from build123d import *

# Parameters (mm, degrees)
SKETCH001_W = 6
SKETCH001_H = 2
SKETCH002_R = 1.6
HOLE_DEPTH  = 2
HOLE_TIPS_R = 1.6


with BuildPart() as part:
    # AdditivePipe: sweep along a path in Sketch
    with BuildLine(Plane.XZ) as additivepipe_path:
        Line((-3, 0), (5.65, 0))
        ThreePointArc((5.65, 0), (6.053202, 0.204318), (6.126879, 0.650289))
        ThreePointArc((6.126879, 0.650289), (5.65, 3.75), (6.126879, 6.849711))
        ThreePointArc((6.126879, 6.849711), (6.053202, 7.295682), (5.65, 7.5))
        Line((5.65, 7.5), (2.5, 7.5))
        ThreePointArc((2.5, 7.5), (2.401942, 7.49029), (2.307692, 7.461538))
        ThreePointArc((2.307692, 7.461538), (0, 7), (-2.307692, 7.461538))
    # Sketch001 → AdditivePipe (sweep)
    with BuildSketch(Plane.YZ):
        with Locations((0, -1)):
            Rectangle(SKETCH001_W, SKETCH001_H)
    sweep(path=additivepipe_path.line)

    # Sketch002 (on DatumPlane) → Hole (cut)
    with BuildSketch(Plane.XY.offset(-2)):
        Circle(SKETCH002_R)
    extrude(amount=HOLE_DEPTH, mode=Mode.SUBTRACT)

    # Hole tips → Hole tip 1 section 0
    with BuildSketch(Plane.XY, mode=Mode.PRIVATE) as hole_tip_1_s0:
        Circle(HOLE_TIPS_R)
    loft([hole_tip_1_s0.sketch, Vertex(0, 0, 0.961377)], mode=Mode.SUBTRACT)


solid = part.part
Design review of the part built by this model. Coordinates are the model's own, in mm. A direction names the side the tool comes from. Give positions to 0.01 mm unless a question says otherwise; leave off trailing zeros. Write each loop counter-clockwise with the first axis right and the second up, starting at its lowest first coordinate (ties: lowest second). Pieces come first, ordered by that corner, then holes. Notation, with made-up numbers: M 2.25,37.5 L 32.25,37.5 A13 ccw 32.25,56.5 Z; hole C -28.5,53.25 d4. An arc over 180 degrees is marked long. Return JSON: item names as keys, results as strings. Group by question number.
Item 1: Take a section at B-B (x = 0). Give the boundary of the cut face in (y, z), plus the area to 3 significant figures.
Item 2: Take a section at A-A (y = 0). Give the boundary of the cut face in (x, z), plus the area to 3 significant figures.
Item 3: Wall thickness on line 1 along Y through (x, z) = (0, -1.1); line 2 along Z through (x, y) = (2.75, 1.5); line 3 along Y through (x, z) = (-0.75, -0.5): over which ranges is each line inside the solid? List them lowest first.
Item 4: The part is to be moulded in two halves that separate along Z. For faces 1 (the flat face through (2, 0, -2)), 2 (the cylindrical face through (-1.27, -0.97, -1.01)), 3 (the flat face through (4, 0, 7.5)), say which applies: pulls with the +Z half, pulls with the -Z half, needs draft (parallel to the pull), parting line crosses it, or undercut.
Item 5: Take a section at C-C (z = -1). Give the boundary of the cut face in (x, y), plus the area to 3 significant figures.
Item 6: Clearance check with a flat-ended pin moving along its axis: pin 1 Ø6 at (x, z) = (2.5, 0.5) entering from +Y. State where the tip first meets the part, or that it passes through.
Item 7: Tool access review of faces 4 (the flat face through (2, 0, 0)), 5 (the flat face through (-1.918, -0.042, 8.398)), 6 (the cylindrical face through (0, 0, 7)): name each direction out of +Z, -Z, +X, -X, +Y, -Y from which nothing blocks a thin tool from reaching the whole face with its end or side.
Item 8: Take a section at D-D (x = 2.75). Give the boundary of the cut face in (y, z), plus the area to 3 significant figures.
Return value:
{
 "1": {"outline": "M -3,-2 L -1.6,-2 L -1.6,0 L -3,0 Z; M -3,7 L 3,7 L 3,9 L -3,9 Z; M 1.6,-2 L 3,-2 L 3,0 L 1.6,0 Z", "area": "17.6 mm2"},
 "2": {"outline": "M -3,-2 L -1.6,-2 L -1.6,0 L -3,0 Z; M -2.31,7.46 A6 ccw 2.31,7.46 A0.5 cw 2.5,7.5 L 5.65,7.5 A0.5 cw 6.13,6.85 A10.31 ccw 6.13,0.65 A0.5 cw 5.65,0 L 1.6,0 L 1.6,-2 L 5.65,-2 A2.5 ccw 8.03,1.25 A8.31 cw 8.03,6.25 A2.5 ccw 5.65,9.5 L 2.5,9.5 A2.5 ccw 1.54,9.31 A4 cw -1.54,9.31 Z", "area": "48.9 mm2"},
 "3": {"line 1": "y = -3 to -1.6, 1.6 to 3", "line 2": "z = -2 to 0, 7.5 to 9.5", "line 3": "y = -3 to -1.41, 1.41 to 3"},
 "4": {"face 1": "pulls with the -Z half", "face 2": "needs draft", "face 3": "undercut"},
 "5": {"outline": "M -3,-3 L 7.65,-3 L 7.65,3 L -3,3 Z; hole C 0,0 d3.2", "area": "55.9 mm2"},
 "6": {"pin 1": "stops at y = 3"},
 "7": {"face 4": "-X, +Y, -Y", "face 5": "+Z, -X, +Y, -Y", "face 6": "+Y, -Y"},
 "8": {"outline": "M -3,-2 L 3,-2 L 3,0 L -3,0 Z; M -3,7.5 L 3,7.5 L 3,9.5 L -3,9.5 Z", "area": "24.0 mm2"}
}
